Verification items for the finished model (mm, model axes). Face numbers are marked on the shaded views. A direction names the side the tool comes from. Round coordinates to 2 decimals unless told otherwise and drop trailing zeros. Order: outer loops, then holes, each group sorted by start corner. A loop starts at its lowest first (then second) coordinate and runs counter-clockwise, first axis right, second up. Notation, with made-up numbers: M 41.5,17.5 L 61.5,17.5 A23 cw 61.5,32.5 Z; hole C -15.75,32 d2. An arc over 180 degrees is marked long. Use one line per item in the form item = value. Start each with the question number.
Item 1: Go/stop test with flat-tipped pins: pin 1 Ø3.5 at (y, z) = (1.5, -4) entering from -X; pin 2 Ø5 at (x, z) = (5.5, 2.5) entering from +Y; pin 3 Ø1.4 at (x, z) = (2.5, -1.5) entering from +Y. Record where each tip stops, or that it passes through.
Item 2: Cross-section at C-C on y = 2.75. Enter the section's corners in (x, z), then the cut area to 3 significant figures.
Item 3: Cross-section at D-D on y = -1.75. Enter the section's corners in (x, z), then the cut area to 3 significant figures.
Item 4: Cross-section at A-A on z = 0. Enter the section's corners in (x, y).
Item 5: Thickness scan on probe 1 along Z at (x, y) = (10, -1.5); probe 2 along X at (y, z) = (-2.1, 0); probe 3 along X at (y, z) = (-0.25, 1). Record the ranges inside material, lowest first. Write a range as [from, to].
Item 6: Cross-section at B-B on x = 8. Enter the section's corners in (y, z), then the cut area to 3 significant figures.
Item 7: Release check for a two-part mould opening along Z. For the marked faces 1, 2 and 3 record: +Z half, -Z half, draft (parallel to the pull), parting line (faces both ways), or undercut.
Item 8: Tool access check on the marked faces 4, 5 and 6. Record the directions out of +Z, -Z, +X, -X, +Y, -Y that give a thin tool (end or side, any length) a straight path to the whole face; none if there is none.
from build123d import *

# Parameters (mm, degrees)
BOSS_EXTRUDE1_DEPTH     = 16
SKETCH2_R               = 3
CUT_EXTRUDE1_DEPTH      = 18
SKETCH3_R               = 4
CUT_EXTRUDE2_DEPTH      = 1
SKETCH4_R               = 3
CUT_EXTRUDE3_DEPTH      = 14
SKETCH5_W               = 6.803133859
SKETCH5_H               = 10.102230074
CUT_EXTRUDE4_DEPTH      = 6
SKETCH6_W               = 5
SKETCH6_H               = 10
CUT_EXTRUDE5_DEPTH      = 4
SKETCH7_W               = 6.342903926
SKETCH7_H               = 4
CUT_EXTRUDE6_DEPTH      = 4
CUT_EXTRUDE6_DEPTH_BACK = 2


with BuildPart() as part:
    # Sketch1 → Boss-Extrude1 (new body)
    with BuildSketch(Plane(origin=(0, 0, 0), x_dir=(0, 0, -1), z_dir=(1, 0, 0))):
        with BuildLine():
            Line((-2, 4), (-5, 4))
            Line((-5, 4), (-5, -4))
            Line((-5, -4), (5, -4))
            Line((5, -4), (5, 4))
            Line((5, 4), (2, 4))
            ThreePointArc((2, 4), (0, 2), (-2, 4))
        make_face()
    extrude(amount=BOSS_EXTRUDE1_DEPTH)

    # Sketch2 → Cut-Extrude1 (cut)
    with BuildSketch(Plane(origin=(0, 4, 0), x_dir=(1, 0, 0), z_dir=(0, 1, 0))):
        with Locations((5.17622925, 0)):
            Circle(SKETCH2_R)
        with BuildLine():
            Line((5, 5), (0, 5))
            Line((0, 5), (0, -5))
            Line((0, -5), (5, -5))
            ThreePointArc((5, -5), (0.173124539, 0), (5, 5))
        make_face()
    extrude(amount=-CUT_EXTRUDE1_DEPTH, mode=Mode.SUBTRACT)

    # Sketch3 → Cut-Extrude2 (cut)
    with BuildSketch(Plane(origin=(16, 0, 0), x_dir=(0, 0, -1), z_dir=(1, 0, 0))):
        with Locations((0, 4)):
            Circle(SKETCH3_R)
    extrude(amount=-CUT_EXTRUDE2_DEPTH, mode=Mode.SUBTRACT)

    # Sketch4 → Cut-Extrude3 (cut)
    with BuildSketch(Plane(origin=(0, 0, 0), x_dir=(0, 0, -1), z_dir=(1, 0, 0))):
        with Locations((0, 4)):
            Circle(SKETCH4_R)
    extrude(amount=CUT_EXTRUDE3_DEPTH, mode=Mode.SUBTRACT)

    # Sketch5 → Cut-Extrude4 (cut)
    with BuildSketch(Plane(origin=(0, 4, 0), x_dir=(1, 0, 0), z_dir=(0, 1, 0))):
        with Locations((1.598433071, -0.051115037)):
            Rectangle(SKETCH5_W, SKETCH5_H)
    extrude(amount=-CUT_EXTRUDE4_DEPTH, mode=Mode.SUBTRACT)

    # Sketch6 → Cut-Extrude5 (cut)
    with BuildSketch(Plane(origin=(0, 4, 0), x_dir=(1, 0, 0), z_dir=(0, 1, 0))):
        with Locations((7.5, 0)):
            Rectangle(SKETCH6_W, SKETCH6_H)
    extrude(amount=-CUT_EXTRUDE5_DEPTH, mode=Mode.SUBTRACT)

    # Sketch7 → Cut-Extrude6 (cut, two sides)
    with BuildSketch(Plane(origin=(0, 0, 0), x_dir=(1, 0, 0), z_dir=(0, 1, 0))) as cut_extrude6_sk:
        with Locations((7.828548037, 0)):
            Rectangle(SKETCH7_W, SKETCH7_H)
    extrude(amount=CUT_EXTRUDE6_DEPTH, mode=Mode.SUBTRACT)
    extrude(cut_extrude6_sk.sketch, amount=-CUT_EXTRUDE6_DEPTH_BACK, mode=Mode.SUBTRACT)


solid = part.part
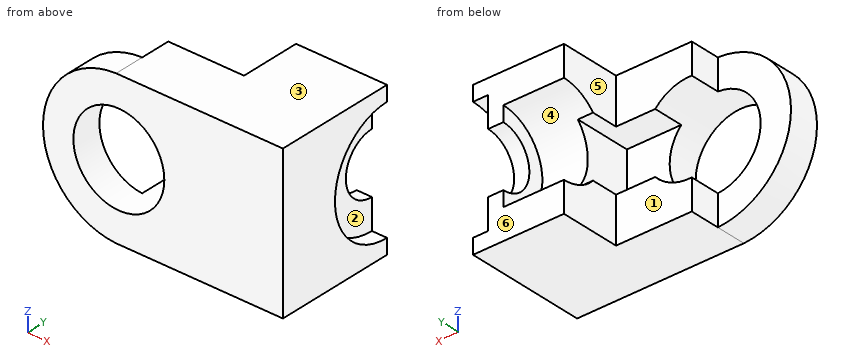
Output values:
q1.pin_1 = 5
q1.pin_2 = 0
q1.pin_3 = -2
q2.outline = M 10,-5 L 16,-5 L 16,-3.8 L 15,-3.8 L 15,-1.56 L 14,-1.56 L 14,-2.73 L 10,-2.73 Z; M 10,2.73 L 14,2.73 L 14,1.56 L 15,1.56 L 15,3.8 L 16,3.8 L 16,5 L 10,5 Z
q2.area = 27.5 mm2
q3.outline = M 5,-5 L 16,-5 L 16,5 L 5,5 L 5,2.99 A3 cw 7.41,2 L 11,2 L 11,-2 L 7.41,-2 A3 cw 5,-2.99 Z
q3.area = 82.6 mm2
q4.outline = M 0.17,-4 L 2.18,-4 L 2.18,-2 L 0.17,-2 Z; M 8.18,-4 L 16,-4 L 16,0 L 15,0 L 15,2 L 14,2 L 14,1 L 11,1 L 11,-2 L 8.18,-2 Z
q5.probe_1 = [-5, -2], [2, 5]
q5.probe_2 = [0.17, 2.18], [8.18, 16]
q5.probe_3 = [11, 16]
q6.outline = M -4,-5 L 0,-5 L 0,-2 L -2,-2 L -2,-1.01 L -4,-1.01 Z; M -4,1.01 L -2,1.01 L -2,2 L 0,2 L 0,5 L -4,5 Z
q6.area = 27.9 mm2
q7.face_1 = draft
q7.face_2 = undercut
q7.face_3 = +Z half
q8.face_4 = -X, +Y
q8.face_5 = +Z, -Z, -X, +Y
q8.face_6 = +Z, -Z, +X, -X, +Y
